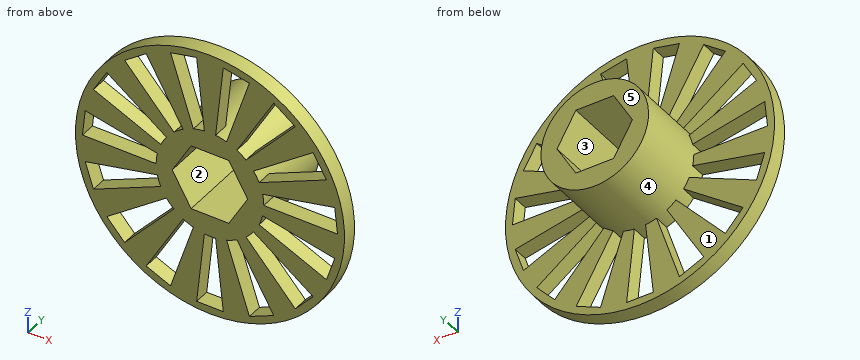
from build123d import *

# Parameters (mm, degrees)
BOSS_EXTRUDE1_DEPTH      = 1
BOSS_EXTRUDE1_DEPTH_BACK = 1
SKETCH1_R                = 17.5
BOSS_EXTRUDE2_START      = -1
SKETCH2_R                = 7
BOSS_EXTRUDE2_DEPTH      = 11


with BuildPart() as part:
    # Sketch1 → Boss-Extrude1 (new, two sides: drawn at the far end of the back side and taken through both)
    with BuildSketch(Plane(origin=(0, 0, 0), x_dir=(1, 0, 0), z_dir=(0, 1, 0)).offset(-BOSS_EXTRUDE1_DEPTH_BACK)):
        with Locations(Location((0, 0, 0), (0, 0, 270))):
            Circle(SKETCH1_R)
        Polygon((3.267901909, 5.66017214), (8.295443306, 14.368129278), (5.126865915, 15.778870824), (2.019674451, 6.21591881), align=None, mode=Mode.SUBTRACT)
        Polygon((0.683177529, 6.5), (1.734219882, 16.5), (-1.734219882, 16.5), (-0.683177529, 6.5), align=None, mode=Mode.SUBTRACT)
        Polygon((5.28757636, 3.841649096), (13.422309222, 9.751878473), (11.101470019, 12.329431536), (4.373306371, 4.857048787), align=None, mode=Mode.SUBTRACT)
        Polygon((6.392980823, 1.358870022), (16.228335934, 3.449439288), (15.156529103, 6.748121527), (5.970753889, 2.658350904), align=None, mode=Mode.SUBTRACT)
        Polygon((6.392980823, -1.358870022), (16.228335934, -3.449439288), (16.590886613, 0), (6.535803817, 0), align=None, mode=Mode.SUBTRACT)
        Polygon((5.28757636, -3.841649096), (13.422309222, -9.751878473), (15.156529103, -6.748121527), (5.970753889, -2.658350904), align=None, mode=Mode.SUBTRACT)
        Polygon((3.267901909, -5.66017214), (8.295443306, -14.368129278), (11.101470019, -12.329431536), (4.373306371, -4.857048787), align=None, mode=Mode.SUBTRACT)
        Polygon((0.683177529, -6.5), (1.734219882, -16.5), (5.126865915, -15.778870824), (2.019674451, -6.21591881), align=None, mode=Mode.SUBTRACT)
        Polygon((-2.019674451, -6.21591881), (-5.126865915, -15.778870824), (-1.734219882, -16.5), (-0.683177529, -6.5), align=None, mode=Mode.SUBTRACT)
        Polygon((-4.373306371, -4.857048787), (-11.101470019, -12.329431536), (-8.295443306, -14.368129278), (-3.267901909, -5.66017214), align=None, mode=Mode.SUBTRACT)
        Polygon((-5.970753889, -2.658350904), (-15.156529103, -6.748121527), (-13.422309222, -9.751878473), (-5.28757636, -3.841649096), align=None, mode=Mode.SUBTRACT)
        Polygon((-6.535803817, 0), (-16.590886613, 0), (-16.228335934, -3.449439288), (-6.392980823, -1.358870022), align=None, mode=Mode.SUBTRACT)
        Polygon((-5.970753889, 2.658350904), (-15.156529103, 6.748121527), (-16.228335934, 3.449439288), (-6.392980823, 1.358870022), align=None, mode=Mode.SUBTRACT)
        Polygon((-4.373306371, 4.857048787), (-11.101470019, 12.329431536), (-13.422309222, 9.751878473), (-5.28757636, 3.841649096), align=None, mode=Mode.SUBTRACT)
        Polygon((-2.019674451, 6.21591881), (-5.126865915, 15.778870824), (-8.295443306, 14.368129278), (-3.267901909, 5.66017214), align=None, mode=Mode.SUBTRACT)
        Polygon((4.907477288, 0), (2.453738644, 4.25), (-2.453738644, 4.25), (-4.907477288, 0), (-2.453738644, -4.25), (2.453738644, -4.25), align=None, mode=Mode.SUBTRACT)
    extrude(amount=BOSS_EXTRUDE1_DEPTH + BOSS_EXTRUDE1_DEPTH_BACK)

    # Sketch2 → Boss-Extrude2 (add)
    with BuildSketch(Plane(origin=(0, 0, 0), x_dir=(1, 0, 0), z_dir=(0, 1, 0)).offset(BOSS_EXTRUDE2_START)):
        with Locations(Location((0, 0, 0), (0, 0, 270))):
            Circle(SKETCH2_R)
        Polygon((4.907477288, 0), (2.453738644, 4.25), (-2.453738644, 4.25), (-4.907477288, 0), (-2.453738644, -4.25), (2.453738644, -4.25), align=None, mode=Mode.SUBTRACT)
    extrude(amount=BOSS_EXTRUDE2_DEPTH)


solid = part.part
Part model, mm, in its own coordinate system. Face numbers are marked on the shaded views. A direction names the side the tool comes from. Coordinates: 2 decimals unless noted, no trailing zeros. Order: outer loops, then holes, each group sorted by start corner. A loop starts at its lowest first (then second) coordinate and runs counter-clockwise, first axis right, second up. Notation, with made-up numbers: M 41.5,54.25 L 85.5,54.25 A12 cw 85.5,73.25 Z; hole C 30,-29.5 d7. An arc over 180 degrees is marked long. Use a Markdown table: item, result.
(1) Tool access for the marked faces 3, 4 and 5: list every direction of +Z, -Z, +X, -X, +Y, -Y with a clear straight run to the whole face (end or side of a thin tool).
A:
| item | result |
|---|---|
| face 3 | +Y, -Y |
| face 4 | +Y |
| face 5 | +Z, -Z, +X, -X, +Y |
(2) Cut at C-C on z = -15. Write the cut outline in (x, y), then the cut area to 3 significant figures.
A:
| item | result |
|---|---|
| outline | M -9.01,-1 L -6.88,-1 L -6.88,1 L -9.01,1 Z; M -4.87,-1 L -1.58,-1 L -1.58,1 L -4.87,1 Z; M 1.58,-1 L 4.87,-1 L 4.87,1 L 1.58,1 Z; M 6.88,-1 L 9.01,-1 L 9.01,1 L 6.88,1 Z |
| area | 21.7 mm^2 |
(3) Cut at D-D on x = 14.5. Write the cut outline in (y, z).
A:
| item | result |
|---|---|
| outline | M -1,-9.8 L 1,-9.8 L 1,-6.46 L -1,-6.46 Z; M -1,-3.08 L 1,-3.08 L 1,0 L -1,0 Z; M -1,3.08 L 1,3.08 L 1,6.46 L -1,6.46 Z; M -1,7.89 L 1,7.89 L 1,9.8 L -1,9.8 Z |
(4) Flat gauge pins, fed straight in: pin 1 (2.5 mm diameter, centred on x = -0.5, y = 6, fed in from +Z); pin 2 (6 mm diameter, centred on y = 6.5, z = -0.5, fed in from +X); pin 3 (17.5 mm diameter, centred on x = 3, z = 8.5, fed in from +Y); pin 4 (2 mm diameter, centred on x = 10, y = -0.5, fed in from +Z). Where does each tip first touch, or does it go through?
A:
| item | result |
|---|---|
| pin 1 | stops at z = 7 |
| pin 2 | stops at x = 7 |
| pin 3 | stops at y = 10 |
| pin 4 | stops at z = 15.01 |
(5) Probe L1, parallel to Z at x = 1.5, y = 9; L2, parallel to X at y = 0, z = -4.5; L3, parallel to Y at x = -6.5, z = 15. List the from-to ranges inside material, lowest first.
A:
| item | result |
|---|---|
| L1 | z = -6.84 to -4.25, 4.25 to 6.84 |
| L2 | x = -16.91 to -15.89, -10.11 to -6.19, -5.36 to 5.36, 6.19 to 10.11, 15.89 to 16.91 |
| L3 | y = -1 to 1 |
(6) Cut at B-B on y = 7.75. Write the cut outline in (x, z).
A:
| item | result |
|---|---|
| outline | C 0,0 d14; hole M -4.91,0 L -2.45,-4.25 L 2.45,-4.25 L 4.91,0 L 2.45,4.25 L -2.45,4.25 Z |
(7) Cut at A-A on x = 0. Write the cut outline in (y, z), then the cut area to 3 significant figures.
A:
| item | result |
|---|---|
| outline | M -1,-17.5 L 1,-17.5 L 1,-16.5 L -1,-16.5 Z; M -1,-7 L 10,-7 L 10,-4.25 L -1,-4.25 Z; M -1,4.25 L 10,4.25 L 10,7 L 1,7 L 1,17.5 L -1,17.5 Z |
| area | 83.5 mm^2 |
(8) Pull direction Z, two halves, no side cores. Call the marked faces 1 and 2: released by +Z, released by -Z, zero draft, split by the parting line, or undercut.
A:
| item | result |
|---|---|
| face 1 | zero draft |
| face 2 | undercut |
